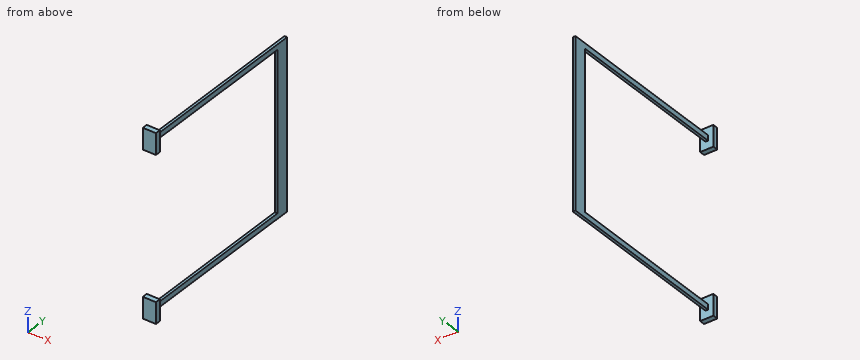
from build123d import *

# Parameters (mm, degrees)
SKETCH_1_W      = 600
SKETCH_1_H      = 50
SKETCH_1_W_2    = 30
SKETCH_1_H_2    = 20
SKETCH_1_W_3    = 20
EXTRUDE_1_DEPTH = 5
SKETCH_1_3_W    = 30
SKETCH_1_3_H    = 20
SKETCH_1_3_W_2  = 20
EXTRUDE_2_DEPTH = 25


with BuildPart() as part:
    # Sketch 1 → Extrude 1 (new, symmetric)
    with BuildSketch(Plane(origin=(0, 0, 0), x_dir=(0, 0, -1), z_dir=(1, 0, 0))):
        Polygon((-300, -25), (-300, 25), (-320, 25), (-320, -655), (-300, -655), align=None)
        Rectangle(SKETCH_1_W, SKETCH_1_H)
        Polygon((320, -655), (320, 25), (300, 25), (300, -25), (300, -655), align=None)
        with Locations((-285, -665)):
            Rectangle(SKETCH_1_W_2, SKETCH_1_H_2)
        with Locations((-310, -665)):
            Rectangle(SKETCH_1_W_3, SKETCH_1_H_2)
        with Locations((-335, -665)):
            Rectangle(SKETCH_1_W_2, SKETCH_1_H_2)
        with Locations((310, -665)):
            Rectangle(SKETCH_1_W_3, SKETCH_1_H_2)
        with Locations((335, -665)):
            Rectangle(SKETCH_1_W_2, SKETCH_1_H_2)
        with Locations((285, -665)):
            Rectangle(SKETCH_1_W_2, SKETCH_1_H_2)
    extrude(amount=EXTRUDE_1_DEPTH, both=True)

    # Sketch 1_3 → Extrude 2 (add, symmetric)
    with BuildSketch(Plane(origin=(0, 0, 0), x_dir=(0, 0, -1), z_dir=(1, 0, 0))):
        with Locations((-335, -665)):
            Rectangle(SKETCH_1_3_W, SKETCH_1_3_H)
        with Locations((-310, -665)):
            Rectangle(SKETCH_1_3_W_2, SKETCH_1_3_H)
        with Locations((-285, -665)):
            Rectangle(SKETCH_1_3_W, SKETCH_1_3_H)
        with Locations((285, -665)):
            Rectangle(SKETCH_1_3_W, SKETCH_1_3_H)
        with Locations((310, -665)):
            Rectangle(SKETCH_1_3_W_2, SKETCH_1_3_H)
        with Locations((335, -665)):
            Rectangle(SKETCH_1_3_W, SKETCH_1_3_H)
    extrude(amount=EXTRUDE_2_DEPTH, both=True)


solid = part.part
Verification items for the finished model (mm, model axes). Give positions to 0.01 mm unless a question says otherwise; leave off trailing zeros. Order: outer loops, then holes, each group sorted by start corner. A loop starts at its lowest first (then second) coordinate and runs counter-clockwise, first axis right, second up. Notation, with made-up numbers: M 21.5,42 L 80.5,42 A26 cw 80.5,81 Z; hole C -16,18 d11. An arc over 180 degrees is marked long. Use one line per item in the form item = value. Start each with the question number.
Q1. Section check C-C (z = 105.5). Enter the section's corners in (x, y), then the cut area to 3 significant figures.
Q2. Section check A-A (z = -282.5). Enter the section's corners in (x, y), then the cut area to 3 significant figures.
Q3. Scan lines: line 1 along Z through (x, y) = (4, -73); line 2 along Y through (x, z) = (3, -108); line 3 along Y through (x, z) = (-18, 316.5). Record each from-to range of solid material in increasing order. Write a range as [from, to].
Q4. Go/stop test with flat-tipped pins: pin 1 Ø8 at (x, y) = (-2.5, -279.5) entering from +Z; pin 2 Ø5 at (x, z) = (-1.5, -63.5) entering from -Y; pin 3 Ø8 at (x, y) = (-2.5, -467) entering from -Z. Record where each tip stops, or that it passes through.
Q5. Section check B-B (y = -349). Enter the section's corners in (x, z), then the cut area to 3 significant figures.
Evaluation:
q1.outline = M -5,-25 L 5,-25 L 5,25 L -5,25 Z
q1.area = 500 mm2
q2.outline = M -25,-675 L 25,-675 L 25,-655 L -25,-655 Z; M -5,-25 L 5,-25 L 5,25 L -5,25 Z
q2.area = 1,500 mm2
q3.line_1 = [-320, -300], [300, 320]
q3.line_2 = [-25, 25]
q3.line_3 = [-675, -655]
q4.pin_1 = 320
q4.pin_2 = -25
q4.pin_3 = -320
q5.outline = M -5,-320 L 5,-320 L 5,-300 L -5,-300 Z; M -5,300 L 5,300 L 5,320 L -5,320 Z
q5.area = 400 mm2
